Geometry: see drawing. Coordinates: mm, zero at the bounding-box minimum. Round coordinates to 2 decimals unless told otherwise and drop trailing zeros. Order: outer loops, then holes, each group sorted by start corner. A loop starts at its lowest first (then second) coordinate and runs counter-clockwise, first axis right, second up. Notation, with made-up numbers: (30.25, 83.5) -> (69.25, 83.5) arc R35 ccw to (69.25, 117.5) -> close; hole circle Ø4 at (23, 39). An arc over 180 degrees is marked (long way). Put each result on its own line as item: value.
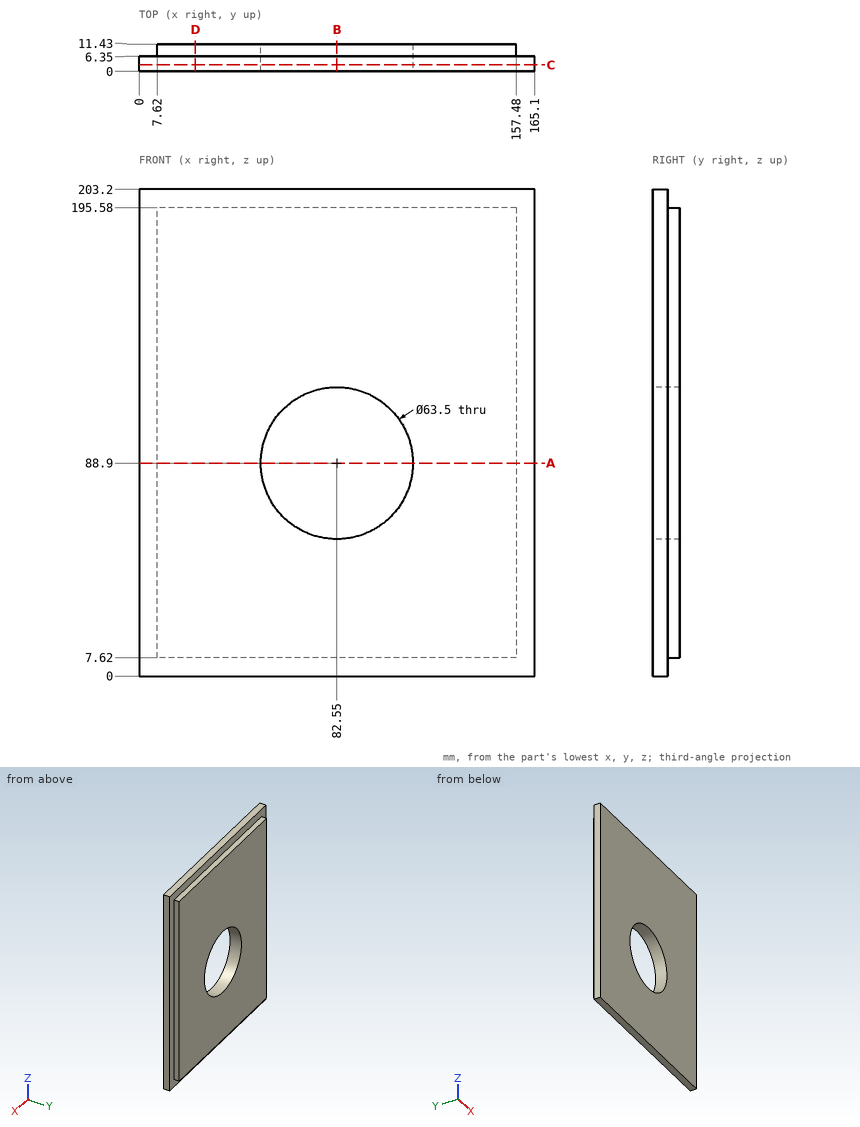
1. Cut plane B-B on x = 82.55. Return loops of the section in (y, z), and give its area (3 significant figures).
Ans:
outline: (0, 0) -> (6.35, 0) -> (6.35, 7.62) -> (11.43, 7.62) -> (11.43, 57.15) -> (0, 57.15) -> close; (0, 120.65) -> (11.43, 120.65) -> (11.43, 195.58) -> (6.35, 195.58) -> (6.35, 203.2) -> (0, 203.2) -> close
area: 1,520 mm²
2. Cut plane C-C on y = 2.75. Return loops of the section in (x, z).
Ans:
outline: (0, 0) -> (165.1, 0) -> (165.1, 203.2) -> (0, 203.2) -> close; hole circle Ø63.5 at (82.55, 88.9)
3. Material intervals for probe 1 along Z at (x, y) = (82.55, 3.5); probe 2 along X at (y, z) = (8, 89); probe 3 along Z at (x, y) = (82.55, 6.5), sorted ascending.
Ans:
probe 1: 0 to 57.15, 120.65 to 203.2
probe 2: 7.62 to 50.8, 114.3 to 157.48
probe 3: 7.62 to 57.15, 120.65 to 195.58
4. Contact query for flat-ended pins moving along their axis: P1, Ø2, axis at y = 9, z = 54.5, coming from the +X side; P2, Ø8, axis at x = 115, z = 150, coming from the -Y side; P3, Ø2.5, axis at y = 8, z = 146.5, coming from the -X side; P4, Ø1.5, axis at x = 92, y = 9.5, coming from the -Z side. Output: stop coordinate, or through.
Ans:
P1: x = 157.48
P2: y = 0
P3: x = 7.62
P4: z = 7.62
5. Cut plane A-A on z = 88.9. Return loops of the section in (x, y).
Ans:
outline: (0, 0) -> (50.8, 0) -> (50.8, 11.43) -> (7.62, 11.43) -> (7.62, 6.35) -> (0, 6.35) -> close; (114.3, 0) -> (165.1, 0) -> (165.1, 6.35) -> (157.48, 6.35) -> (157.48, 11.43) -> (114.3, 11.43) -> close
6. Cut plane D-D on x = 23.5. Return loops of the section in (y, z).
Ans:
outline: (0, 0) -> (6.35, 0) -> (6.35, 7.62) -> (11.43, 7.62) -> (11.43, 195.58) -> (6.35, 195.58) -> (6.35, 203.2) -> (0, 203.2) -> close
